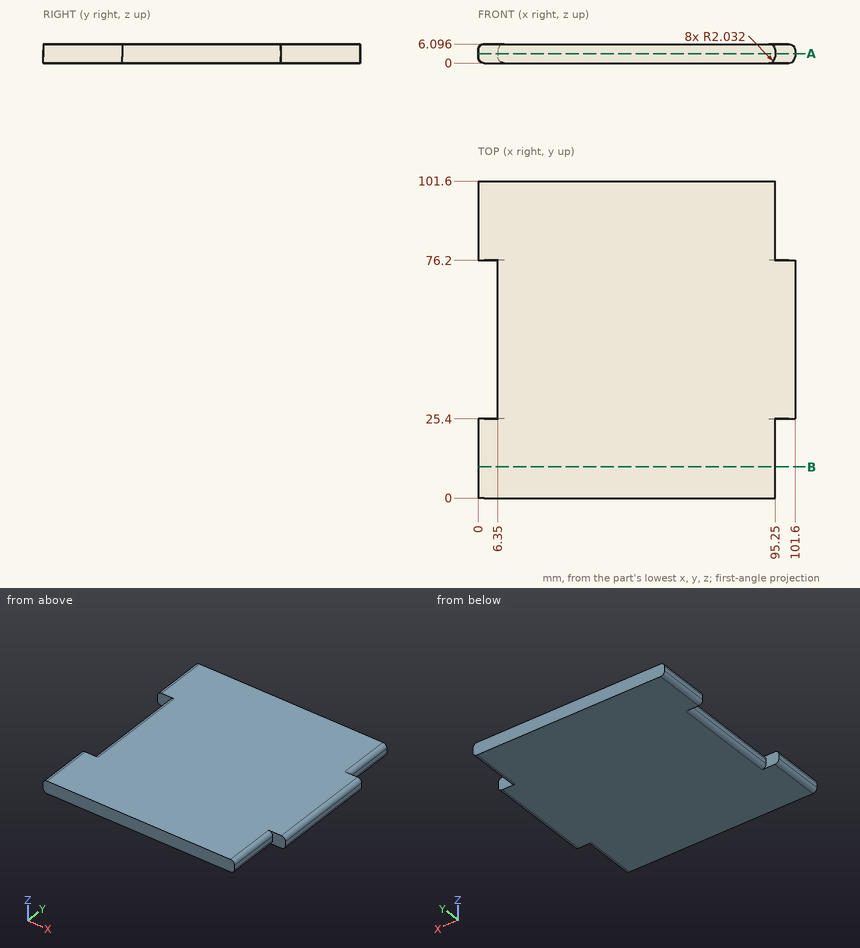
The figure shows three views and two pictorial views of one solid part (mm, origin at its lowest corner). Answer the questions. Coordinates: 2 decimals unless noted, no trailing zeros. Loops run counter-clockwise (first coordinate to the right, second up) from the corner with the lowest first, then second, coordinate; pieces in that order, holes last.
1) Find the intervals of material crossed by L1, parallel to X at y = 56.5, z = 3.75; L2, parallel to Z at x = 94, y = 18.5, in increasing order.
2) Flat-ended cylindrical pins translate along their axes: pin 1 Ø1.6 at (y, z) = (14, 2.5) entering from +X; pin 2 Ø1.8 at (x, z) = (99, 2) entering from -Y; pin 3 Ø1.6 at (y, z) = (52.5, 3) entering from -X. Find the tip coordinate at first contact, or state that the pin passes through.
3) Find section B-B on y = 10. Write down the section's boundary in (x, z).
4) Find section A-A on z = 3. Write down the section's boundary in (x, y), then the cut area to 3 significant figures.
Values:
1. L1: x = 6.35 to 101.6
1. L2: z = 0.16 to 5.94
2. pin 1: stops at x = 95.25
2. pin 2: stops at y = 25.4
2. pin 3: stops at x = 6.35
3. outline: (0, 2.03) arc R2.03 ccw to (2.03, 0) - (93.22, 0) arc R2.03 ccw to (95.25, 2.03) - (95.25, 4.06) arc R2.03 ccw to (93.22, 6.1) - (2.03, 6.1) arc R2.03 ccw to (0, 4.06) - close
4. outline: (0, 0) - (95.25, 0) - (95.25, 25.4) - (101.6, 25.4) - (101.6, 76.2) - (95.25, 76.2) - (95.25, 101.6) - (0, 101.6) - (0, 76.2) - (6.35, 76.2) - (6.35, 25.4) - (0, 25.4) - close
4. area: 9,680 mm2
